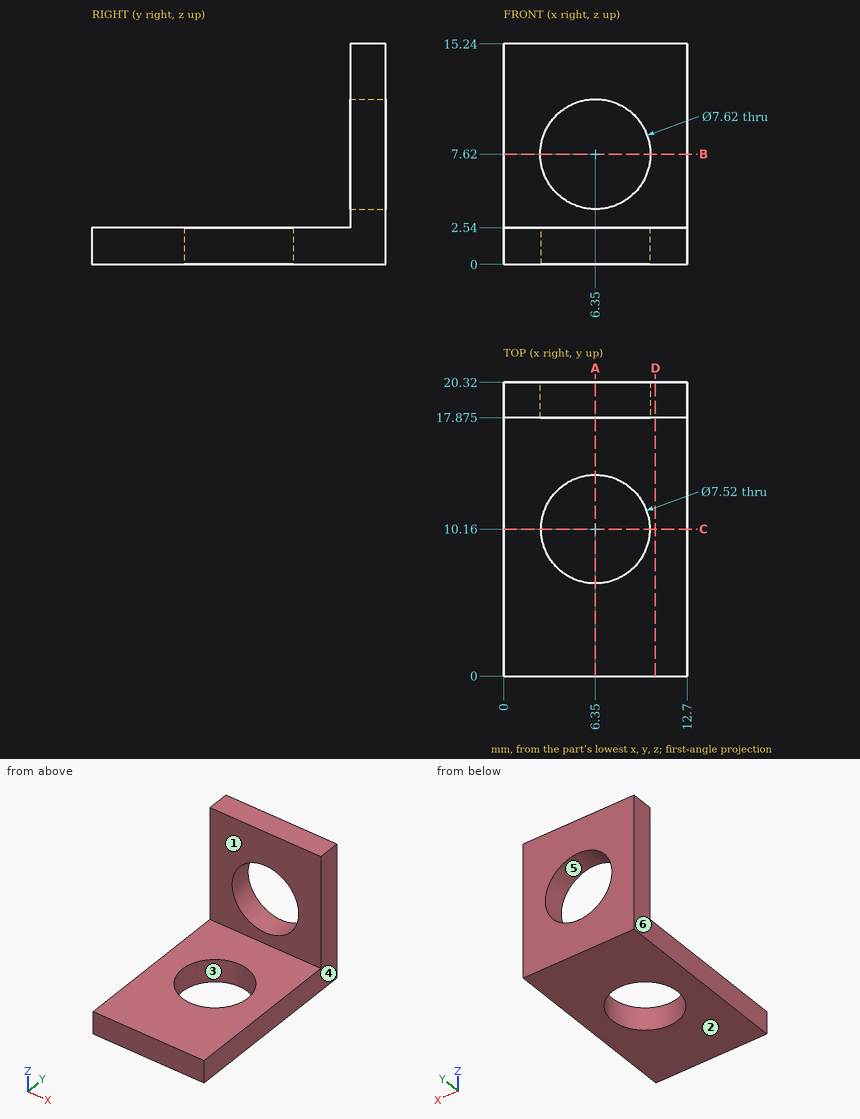
Geometry: see drawing. Coordinates: mm, zero at the bounding-box minimum. A direction names the side the tool comes from. Coordinates: 2 decimals unless noted, no trailing zeros. Order: outer loops, then holes, each group sorted by start corner. A loop starts at its lowest first (then second) coordinate and runs counter-clockwise, first axis right, second up. Notation, with made-up numbers: (3.5, 71) - (52.5, 71) arc R17 cw to (52.5, 88) - close; hole circle Ø5 at (33.5, 69). An arc over 180 degrees is marked (long way). Return JSON: item names as keys, results as strings.
Q1. First-contact query: pin 1 (1 mm diameter, centred on x = 2, y = 15, fed in from +Z); pin 2 (6.5 mm diameter, centred on x = 4, z = 8, fed in from -Y) (1 decimal). Flat tips, straight axial feed; report the tip coordinate or a pass-through.
The answers:
{"pin 1": "stops at z = 2.54", "pin 2": "stops at y = 17.9"}
Q2. Cut plane A-A (x = 6.35). Return loops of the section in (y, z) (1 decimal).
The answers:
{"outline": "(0, 0) - (6.4, 0) - (6.4, 2.5) - (0, 2.5) - close; (13.9, 0) - (20.3, 0) - (20.3, 3.8) - (17.9, 3.8) - (17.9, 2.5) - (13.9, 2.5) - close; (17.9, 11.4) - (20.3, 11.4) - (20.3, 15.2) - (17.9, 15.2) - close"}
Q3. Cut plane D-D (x = 10.5). Return loops of the section in (y, z) (1 decimal).
The answers:
{"outline": "(0, 0) - (20.3, 0) - (20.3, 15.2) - (17.9, 15.2) - (17.9, 2.5) - (0, 2.5) - close"}
Q4. Ray query, probe 1 along Y at (x, z) = (6.35, 1.25); probe 2 along Z at (x, y) = (6.35, 18.55); probe 3 along X at (y, z) = (19.65, 7.62). Return the intervals inside material, ascending.
The answers:
{"probe 1": "y = 0 to 6.4, 13.92 to 20.32", "probe 2": "z = 0 to 3.81, 11.43 to 15.24", "probe 3": "x = 0 to 2.54, 10.16 to 12.7"}
Q5. Draft query along X for the marked faces 3, 4, 5 and 6. Return one class per face: +X half, -X half, draft (parallel to the pull), parting line (faces both ways), or undercut.
The answers:
{"face 3": "undercut", "face 4": "+X half", "face 5": "undercut", "face 6": "-X half"}
Q6. Cut plane C-C (y = 10.16). Return loops of the section in (x, z).
The answers:
{"outline": "(0, 0) - (2.59, 0) - (2.59, 2.54) - (0, 2.54) - close; (10.11, 0) - (12.7, 0) - (12.7, 2.54) - (10.11, 2.54) - close"}
Q7. Access query for the marked faces 1 and 2. Directions: +Z, -Z, +X, -X, +Y, -Y. A direction counts if a zero-diameter tool reaches every point of the face in a straight line with its end or side. Return the directions, or none.
The answers:
{"face 1": "+Z, +X, -X, -Y", "face 2": "-Z, +X, -X, +Y, -Y"}
Q8. Cut plane B-B (z = 7.62). Return loops of the section in (x, y) (1 decimal), then the cut area to 3 significant figures.
The answers:
{"outline": "(0, 17.9) - (2.5, 17.9) - (2.5, 20.3) - (0, 20.3) - close; (10.2, 17.9) - (12.7, 17.9) - (12.7, 20.3) - (10.2, 20.3) - close", "area": "12.4 mm2"}
